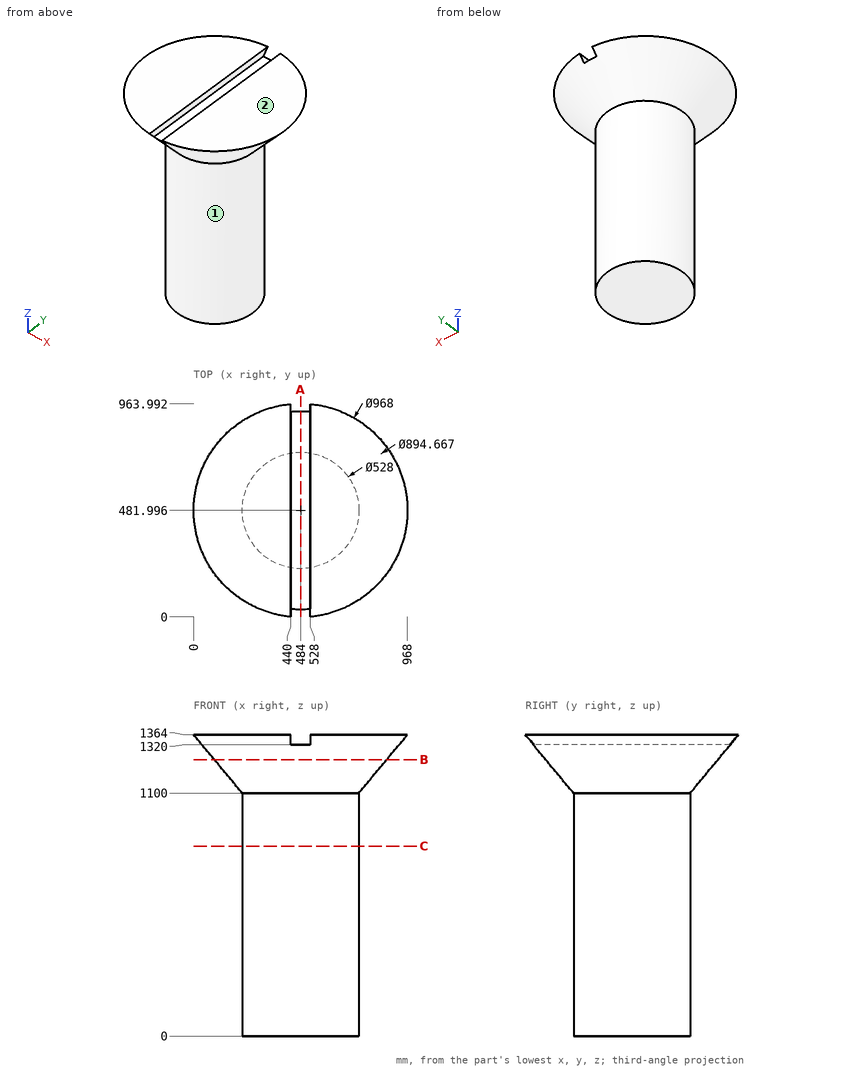
Could you check a few things on this drawing? It's one solid part, dimensions in mm from its lowest x, y, z. A direction names the side the tool comes from. Give positions to 0.01 mm unless a question says otherwise; leave off trailing zeros. Order: outer loops, then holes, each group sorted by start corner. A loop starts at its lowest first (then second) coordinate and runs counter-clockwise, first axis right, second up. Notation, with made-up numbers: (44.25, -20) - (72.25, -20) arc R19 cw to (72.25, -3) - close; hole circle Ø1 at (-1, 71.25). An arc over 180 degrees is marked (long way). One line per item, written item: value. Start each with the question number.
1. If I drill on probe 1 along Z at (x, y) = (509, 481.5); probe 2 along Z at (x, y) = (665.5, 838); probe 3 along X at (y, z) = (700, 313.5) (1 decimal), over which ranges is the centre line in solid material (lowest first)?
2. Imagine slicing it at C-C on z = 859.5. List the corners of the cut face in (x, y) for me, plus the area to 3 significant figures.
3. For the marked faces 1 and 2, which set-ups out of +Z, -Z, +X, -X, +Y, -Y let a thin tool reach every point of the face, with its end or its side?
4. Imagine slicing it at A-A on x = 484. List the corners of the cut face in (y, z) for me, plus the area to 3 significant figures.
5. Imagine slicing it at B-B on z = 1252. List the corners of the cut face in (x, y) for me.
6. For P1, Ø8, axis at y = 519, z = 1170.5, coming from the -X side; P2, Ø10, axis at x = 693.5, y = 362.5, coming from the -Z side; P3, Ø10, axis at y = 394.5, z = 260.5, coming from the -X side; P4, Ø6, axis at y = 450.5, z = 237.5, coming from the -X side, each with a flat end and sliding along its axis, tell me the tip position at first contact or that it passes through.
Values:
1. probe 1: 0 to 1320
1. probe 2: 1262.72 to 1364
1. probe 3: 335.1 to 632.9
2. outline: circle Ø528 at (484, 482)
2. area: 219,000 mm²
3. face 1: -Z
3. face 2: +Z, +X, -X, +Y, -Y
4. outline: (34.66, 1320) - (218, 1100) - (218, 0) - (746, 0) - (746, 1100) - (929.33, 1320) - close
4. area: 737,000 mm²
5. outline: circle Ø781.33 at (484, 482)
6. P1: x = 159.99
6. P2: z = 0
6. P3: x = 233.22
6. P4: x = 221.54
